```python
from build123d import *

# Parameters (mm, degrees)
SKETCH1_W             = 45
SKETCH1_H             = 73
SKETCH1_W_2           = 34.5
SKETCH1_H_2           = 29
BOSS_EXTRUDE1_DEPTH   = 4
BOSS_EXTRUDE2_DEPTH   = 20
SKETCH6_W             = 22
SKETCH6_H             = 4
BOSS_EXTRUDE3_DEPTH   = 22
F_6_CLEARANCE_HOLE1_D = 4.3053
F_6_CLEARANCE_HOLE2_D = 4.3053
M2_CLEARANCE_HOLE1_D  = 2.6
RIB3_REACH            = 63.078
SKETCH12_WALL_W       = 140.31113285
SKETCH12_WALL_H       = 3
RIB4_REACH            = 63.078
SKETCH13_WALL_W       = 143.310838334
SKETCH13_WALL_H       = 3
FILLET2_R             = 2
FILLET3_R             = 5
FILLET4_R             = 10


with BuildPart() as part:
    # Sketch1 → Boss-Extrude1 (new body)
    with BuildSketch(Plane(origin=(0, 0, 0), x_dir=(1, 0, 0), z_dir=(0, 1, 0))):
        Rectangle(SKETCH1_W, SKETCH1_H)
        Rectangle(SKETCH1_W_2, SKETCH1_H_2, mode=Mode.SUBTRACT)
    extrude(amount=BOSS_EXTRUDE1_DEPTH)

    # Sketch2 → Boss-Extrude2 (add, symmetric)
    with BuildSketch(Plane.XY):
        Polygon((-22.5, 4), (-22.5, 10), (-41.5, 10), (-41.5, 6), (-26.5, 6), (-26.5, 0), (-22.5, 0), align=None)
    boss_extrude2 = extrude(amount=BOSS_EXTRUDE2_DEPTH, both=True)

    # Sketch6 → Boss-Extrude3 (add)
    with BuildSketch(Plane(origin=(0, 4, 0), x_dir=(1, 0, 0), z_dir=(0, 1, 0))):
        with Locations((0, -16.5)):
            Rectangle(SKETCH6_W, SKETCH6_H)
    boss_extrude3 = extrude(amount=BOSS_EXTRUDE3_DEPTH)

    # #6 Clearance Hole1 (through all)
    with Locations(Plane(origin=(0, 6, 0), x_dir=(-1, 0, 0), z_dir=(0, -1, 0))):
        with Locations((37.175, -9.779), (37.175, 9.779)):
            f_6_clearance_hole1 = Hole(F_6_CLEARANCE_HOLE1_D / 2)

    # #6 Clearance Hole2 (through all)
    with Locations(Plane(origin=(0, 4, 0), x_dir=(1, 0, 0), z_dir=(0, 1, 0))):
        with Locations((-13.470384182, -32.175), (13.470384182, -32.175)):
            f_6_clearance_hole2 = Hole(F_6_CLEARANCE_HOLE2_D / 2)

    # M2 Clearance Hole1 (through all)
    with Locations(Plane.XY.offset(18.5)):
        with Locations((6, 18.7), (-6, 18.7)):
            m2_clearance_hole1 = Hole(M2_CLEARANCE_HOLE1_D / 2)

    # Sketch12 wall → Rib3 (add, up to next)
    with BuildSketch(Plane(origin=(-34, 3, 0), x_dir=(-0.928476690885, 0.371390676354, 0), z_dir=(-0.371390676354, -0.928476690885, 0)), mode=Mode.PRIVATE) as rib3_sk1:
        Rectangle(SKETCH12_WALL_W, SKETCH12_WALL_H)
    rib3_tool1 = extrude(rib3_sk1.sketch, amount=-RIB3_REACH, mode=Mode.PRIVATE) - part.part
    rib3 = rib3_tool1.solids().sort_by_distance((-34, 3, 0))[0]
    add(rib3)

    # Sketch13 wall → Rib4 (add, up to next)
    with BuildSketch(Plane(origin=(0, 13, 21.775732109), x_dir=(0, 0.939692620782, -0.342020143335), z_dir=(0, 0.342020143335, 0.939692620782)), mode=Mode.PRIVATE) as rib4_sk1:
        Rectangle(SKETCH13_WALL_W, SKETCH13_WALL_H)
    rib4_tool1 = extrude(rib4_sk1.sketch, amount=-RIB4_REACH, mode=Mode.PRIVATE) - part.part
    rib4 = rib4_tool1.solids().sort_by_distance((0, 13, 21.775732109))[0]
    add(rib4)

    # Mirror1: Boss-Extrude3, #6 Clearance Hole2, M2 Clearance Hole1, Rib4 across plane
    add(boss_extrude3.mirror(Plane.XY))
    add(f_6_clearance_hole2.mirror(Plane.XY), mode=Mode.SUBTRACT)
    add(m2_clearance_hole1.mirror(Plane.XY), mode=Mode.SUBTRACT)
    add(rib4.mirror(Plane.XY))

    # Mirror4: Boss-Extrude2, #6 Clearance Hole1, Rib3 across plane
    add(boss_extrude2.mirror(Plane(origin=(0, 0, 0), x_dir=(0, 0, 1), z_dir=(1, 0, 0))))
    add(f_6_clearance_hole1.mirror(Plane(origin=(0, 0, 0), x_dir=(0, 0, 1), z_dir=(1, 0, 0))), mode=Mode.SUBTRACT)
    add(rib3.mirror(Plane(origin=(0, 0, 0), x_dir=(0, 0, 1), z_dir=(1, 0, 0))))

    # Fillet2
    fillet2_edges = [part.edges().sort_by_distance(p)[0] for p in [
        (6.25, 4, 18.5),
        (1.5, 4, 21.775732109),
        (-1.5, 4, 21.775732109),
        (-11, 4, -16.5),
        (-6.25, 4, -18.5),
        (11, 4, -16.5),
        (6.25, 4, -18.5),
        (1.5, 4, -21.775732109),
        (-1.5, 4, -21.775732109),
        (22.5, 4, 0),
        (22.5, 10, 0),
        (-22.5, 4, 0),
        (-22.5, 10, 0),
        (-11, 4, 16.5),
        (-6.25, 4, 18.5),
        (11, 4, 16.5),
    ]]
    fillet(fillet2_edges, radius=FILLET2_R)

    # Fillet3
    fillet3_edges = [part.edges().sort_by_distance(p)[0] for p in [
        (-11, 26, -16.5),
        (11, 26, -16.5),
        (41.5, 8, 20),
        (41.5, 8, -20),
        (-41.5, 8, -20),
        (-41.5, 8, 20),
        (-11, 26, 16.5),
        (11, 26, 16.5),
        (-22.5, 2, -36.5),
        (22.5, 2, -36.5),
        (22.5, 2, 36.5),
        (-22.5, 2, 36.5),
    ]]
    fillet(fillet3_edges, radius=FILLET3_R)

    # Fillet4
    # the kernel refuses this fillet: 10 mm, written as the material it adds along each edge
    with BuildSketch(Plane(origin=(22.5, 4, 20), x_dir=(1, 0, 0), z_dir=(0, -1, 0))) as fillet4_piece_1:
        with BuildLine():
            CenterArc((10, 8), FILLET4_R, 180, 53.130102354)
            Line((0, 8), (0, 0))
            Line((0, 0), (4, 0))
        make_face()
    extrude(amount=4)
    with BuildSketch(Plane(origin=(22.5, 0, -20), x_dir=(0, 0, -1), z_dir=(0, 1, 0))) as fillet4_piece_2:
        with BuildLine():
            CenterArc((8, -10), FILLET4_R, 90, 53.130102354)
            Line((0, -4), (0, 0))
            Line((0, 0), (8, 0))
        make_face()
    extrude(amount=4)
    with BuildSketch(Plane(origin=(-22.5, 0, -20), x_dir=(0, 0, -1), z_dir=(0, 1, 0))) as fillet4_piece_3:
        with BuildLine():
            CenterArc((8, 10), FILLET4_R, 216.869897646, 53.130102354)
            Line((0, 4), (0, 0))
            Line((0, 0), (8, 0))
        make_face()
    extrude(amount=4)
    with BuildSketch(Plane(origin=(-22.5, 4, 20), x_dir=(-1, 0, 0), z_dir=(0, -1, 0))) as fillet4_piece_4:
        with BuildLine():
            CenterArc((10, -8), FILLET4_R, 126.869897646, 53.130102354)
            Line((0, -8), (0, 0))
            Line((0, 0), (4, 0))
        make_face()
    extrude(amount=4)


solid = part.part
```
For this review, take the finished solid that the model builds, in its own axes (mm). A direction names the side the tool comes from. Round coordinates to 2 decimals unless told otherwise and drop trailing zeros. Loops run counter-clockwise (first coordinate to the right, second up) from the corner with the lowest first, then second, coordinate; pieces in that order, holes last.
(1) Wall thickness on line 1 along X through (y, z) = (18.7, -17.5); line 2 along Z through (x, y) = (10, 21); line 3 along Y through (x, z) = (16.5, -25): over which ranges is each line inside the solid? List them lowest first.
Returned:
line 1: x = -11 to -7.3, -4.7 to 4.7, 7.3 to 11
line 2: z = -18.5 to -14.5, 14.5 to 18.5
line 3: y = 0 to 4
(2) We need section C-C (z = -23). Give the boundary of the cut face in (x, y).
Returned:
outline: (-23.84, 0) - (23.84, 0) - (23.84, 4) - (3.5, 4) arc R2 cw to (1.5, 6) - (1.5, 9.64) - (-1.5, 9.64) - (-1.5, 6) arc R2 cw to (-3.5, 4) - (-23.84, 4) - close
(3) Tool access review of faces 1 (the flat face through (1.5, 12, 21)), 2 (the flat face through (-1.5, 12, -21)), 3 (the flat face through (-26.5, 3, 11)), 4 (the flat face through (-18, 4, -1)): name each direction out of +Z, -Z, +X, -X, +Y, -Y from which nothing blocks a thin tool from reaching the whole face with its end or side.
Returned:
face 1: +Z, +Y
face 2: -Z, +Y
face 3: +Z, -X, -Y
face 4: +Y
(4) We need section B-B (y = 18.7). State how many separate pieces and enclosed holes the cut face has, plus the area to 3 significant figures.
Returned:
separate pieces: 6
enclosed holes: 0
area: 142 mm2
(5) Mouldability with a two-part tool opening along Z and no side actions: class faces 5 (the cylindrical face through (35.122, 8.028, 9.132)), 6 (the flat face through (-0.02, 12.96, -21.79)), 7 (the flat face through (-1.5, 12, 21)) as released by +Z, released by -Z, zero draft, split by the parting line, or undercut.
Returned:
face 5: undercut
face 6: released by -Z
face 7: zero draft
(6) Clearance check with flat-ended pins moving along their axes: P1, Ø3, axis at y = 14, z = -17, coming from the +X side; P2, Ø3, axis at y = 15, z = -22, coming from the +X side; P3, Ø4.5, axis at x = -37.5, z = 11.5, coming from the -Y side; P4, Ø2.5, axis at x = -6, y = 18.7, coming from the +Z side. State where each tip first meets the part, or that it passes through.
Returned:
P1: stops at x = 11
P2: stops at x = 1.5
P3: stops at y = 6
P4: passes through
(7) We need section A-A (z = 6). Give the boundary of the cut face in (x, y), plus the area to 3 significant figures.
Returned:
outline: (-41.5, 6) - (-26.5, 6) - (-26.5, 0) - (-17.25, 0) - (-17.25, 4) - (-20.5, 4) arc R2 cw to (-22.5, 6) - (-22.5, 8) arc R2 ccw to (-24.5, 10) - (-41.5, 10) - close; (17.25, 0) - (26.5, 0) - (26.5, 6) - (41.5, 6) - (41.5, 10) - (24.5, 10) arc R2 ccw to (22.5, 8) - (22.5, 6) arc R2 cw to (20.5, 4) - (17.25, 4) - close
area: 242 mm2
